The listing builds one solid part. Answer for the finished solid, in the listing's coordinates (mm). A direction names the side the tool comes from. Round coordinates to 2 decimals unless told otherwise and drop trailing zeros. Write each loop counter-clockwise with the first axis right and the second up, starting at its lowest first coordinate (ties: lowest second). Pieces come first, ordered by that corner, then holes.
from build123d import *

# Parameters (mm, degrees)
BOSS_EXTRUDE1_DEPTH = 3
SKETCH2_R           = 37.5
CUT_EXTRUDE1_DEPTH  = 3
SKETCH3_W           = 4
SKETCH3_H           = 15
BOSS_EXTRUDE4_DEPTH = 3


with BuildPart() as part:
    # Sketch1 → Boss-Extrude1 (new body)
    with BuildSketch(Plane.XY):
        Polygon((11.337032692, 53.818878563), (0, 0), (-220, 0), (-220, 45), (-121.162967308, 73.986910298), align=None)
        Polygon((-94.409209541, 46.483265917), (-94.409209541, 59.799500594), (-120.476048116, 63.767174765), (-179.409209541, 46.483265917), align=None, mode=Mode.SUBTRACT)
    extrude(amount=-BOSS_EXTRUDE1_DEPTH)

    # Sketch2 → Cut-Extrude1 (cut)
    with BuildSketch(Plane.XY):
        with Locations((-182, -15)):
            Circle(SKETCH2_R)
        with Locations((-40, -15)):
            Circle(SKETCH2_R)
    extrude(amount=-CUT_EXTRUDE1_DEPTH, mode=Mode.SUBTRACT)

    # Sketch3 → Boss-Extrude4 (add)
    with BuildSketch(Plane.XY):
        Polygon((-206.731962629, 53.05972607), (-205.606257375, 49.221394704), (-220, 45), (-220, 30), (-224, 30), (-224, 45), (-224, 47.99535863), (-221.125705254, 48.838331367), align=None)
        Polygon((-192.338220004, 57.281120774), (-191.21251475, 53.442789407), (-176.818772125, 57.664184111), (-177.944477379, 61.502515478), align=None)
        Polygon((-121.437734985, 78.074804512), (-106.694649955, 75.830736536), (-107.296563448, 71.876283331), (-121.162967308, 73.986910298), (-133.63754425, 70.328368222), (-134.763249504, 74.166699588), align=None)
        Polygon((-77.03625092, 71.316385344), (-77.638164413, 67.361932139), (-92.46736393, 69.619107735), (-91.865450438, 73.57356094), align=None)
        Polygon((-3.492166825, 56.076054159), (-2.890253333, 60.030507363), (11.938946184, 57.773331767), (16.003099334, 57.297974706), (15.251132951, 52.994367094), (12.159214944, 38.316491123), (8.245114685, 39.141002591), (11.337032692, 53.818878563), align=None)
        Polygon((-18.321366343, 58.333229755), (-17.719452851, 62.287682959), (-32.548652368, 64.544858556), (-33.15056586, 60.590405351), align=None)
        Polygon((-163.550734754, 65.723910181), (-162.4250295, 61.885578815), (-148.031286875, 66.106973518), (-149.156992129, 69.945304885), align=None)
        Polygon((-47.979765378, 62.847580947), (-47.377851886, 66.802034152), (-62.207051403, 69.059209748), (-62.808964895, 65.104756543), align=None)
        with Locations((-222, 7.5)):
            Rectangle(SKETCH3_W, SKETCH3_H)
        Polygon((5.153196678, 24.463126619), (9.067296937, 23.638615151), (5.97537893, 8.960739179), (2.061278671, 9.785250648), align=None)
    extrude(amount=-BOSS_EXTRUDE4_DEPTH)


solid = part.part
1. Section A-A on x = -159 is taken. Determine the outline of the cut face in (y, z), plus the area to 3 significant figures.
Geometry says:
outline: (14.62, -3) - (46.48, -3) - (46.48, 0) - (14.62, 0) - close; (52.47, -3) - (67.06, -3) - (67.06, 0) - (52.47, 0) - close
area: 139 mm2
2. Section D-D on x = -189 is taken. Determine the outline of the cut face in (y, z), plus the area to 3 significant figures.
Geometry says:
outline: (21.84, -3) - (58.26, -3) - (58.26, 0) - (21.84, 0) - close
area: 109 mm2
3. Given pin 1 (0.9 mm diameter, centred on y = 55.5, z = -1, fed in from -X), flat-ended and moving along its own axis, determine where the tip first touches the part or whether it passes through.
Geometry says:
pin 1: stops at x = -191.95
4. Section B-B on x = -97 is taken. Determine the outline of the cut face in (y, z), plus the area to 3 significant figures.
Geometry says:
outline: (0, -3) - (46.48, -3) - (46.48, 0) - (0, 0) - close; (60.19, -3) - (70.31, -3) - (70.31, 0) - (60.19, 0) - close
area: 170 mm2
5. A tool of negligible diameter and unlimited length cuts with its end or side. For faces 5 (the face through (-107.26, 61.756, -1.479)), 6 (the face through (-128.194, 76.093, -1.479)), from which of +Z, -Z, +X, -X, +Y, -Y can it reach the whole face along a straight path? Write none if from no direction.
Geometry says:
face 5: +Z, -Z
face 6: +Z, -Z, -X, +Y
6. Section C-C on x = -13 is taken. Determine the outline of the cut face in (y, z), plus the area to 3 significant figures.
Geometry says:
outline: (11.02, -3) - (57.52, -3) - (57.52, 0) - (11.02, 0) - close
area: 139 mm2
7. Straight lines are drawn through the part: line 1 along X through (y, z) = (6, -0.4); line 2 along X through (y, z) = (13, -0.45); line 3 along Y through (x, z) = (-171, -2.2). For each, find the intervals that lie inside material, in ascending order.
Geometry says:
line 1: x = -224 to -213.07, -150.93 to -71.07, -8.93 to 1.26
line 2: x = -224 to -206.94, -157.06 to -64.94, -15.06 to 6.83
line 3: y = 20.85 to 46.48, 48.95 to 59.37
8. For a pull along Y with two mould halves and no side action, classify faces 1 (the face through (-149.53, 55.246, -1.479)), 2 (the face through (-102, 40, 0)), 3 (the face through (-181.391, 22.495, -1.479)), 4 (the face through (-185.04, 59.42, -1.48)) as released by +Y, released by -Y, zero draft, split by the parting line, or undercut.
Geometry says:
face 1: undercut
face 2: zero draft
face 3: released by -Y
face 4: released by +Y
